```python
from build123d import *
from build123d.topology import SkipClean

# Parameters (mm, degrees)
FILLET_1_R = 2


with BuildPart() as part:
    # ｽｹｯﾁ1 → 回転1 (revolve)
    with SkipClean():  # the faces are left unmerged after this step: merging them gives an invalid solid
        with BuildSketch(Plane.XY, mode=Mode.PRIVATE) as revolve_1_sk:
            with BuildLine():
                ThreePointArc((41.145537471, 23.155045442), (38.343164799, 26.082487024), (34.436430544, 27.159814398))
                Line((34.436430544, 27.159814398), (34.436430544, 11.915416826))
                ThreePointArc((34.436430544, 11.915416826), (39.826138993, 14.147907163), (42.05862933, 19.537615612))
                ThreePointArc((42.05862933, 19.537615612), (41.826831785, 21.403060285), (41.145537471, 23.155045442))
            make_face()
            with BuildLine():
                Line((34.436430544, 11.915416826), (34.436430544, 27.159814398))
                ThreePointArc((34.436430544, 27.159814398), (26.814231757, 19.537615612), (34.436430544, 11.915416826))
            make_face()
            with BuildLine():
                ThreePointArc((42.05862933, 19.537615612), (39.826138993, 14.147907163), (34.436430544, 11.915416826))
                Line((34.436430544, 11.915416826), (34.436430544, 7.442165664))
                Line((34.436430544, 7.442165664), (34.436430544, 4.442165664))
                Line((34.436430544, 4.442165664), (36.436430544, 4.442165664))
                Line((36.436430544, 4.442165664), (36.436430544, 7.442165664))
                Line((36.436430544, 7.442165664), (41.127456758, 7.442165664))
                Line((41.127456758, 7.442165664), (41.127456758, 11.596223188))
                Line((41.127456758, 11.596223188), (44.380435509, 16.421475002))
                Line((44.380435509, 16.421475002), (44.380435509, 22.787256507))
                Line((44.380435509, 22.787256507), (41.735375917, 24.233678208))
                Line((41.735375917, 24.233678208), (41.145537471, 23.155045442))
                ThreePointArc((41.145537471, 23.155045442), (41.826831785, 21.403060285), (42.05862933, 19.537615612))
            make_face()
        revolve(revolve_1_sk.sketch.rotate(Axis((34.436430544, 27.159814398, 0), (0, -1, 0)), 180), axis=Axis((34.436430544, 27.159814398, 0), (0, -1, 0)))

    # ﾌｨﾚｯﾄ1
    fillet_1_edges = [part.edges().sort_by_distance(p)[0] for p in [
        (44.380435509, 22.787256507, 0),
        (41.127456758, 11.596223188, 0),
    ]]
    fillet(fillet_1_edges, radius=FILLET_1_R)


solid = part.part
```
Can you work these out from the model? Positions are in its coordinate system, mm. A direction names the side the tool comes from. Round coordinates to 2 decimals unless told otherwise and drop trailing zeros. Loops run counter-clockwise (first coordinate to the right, second up) from the corner with the lowest first, then second, coordinate; pieces in that order, holes last. Notation, with made-up numbers: M 41.5,57.5 L 95.5,57.5 A19 cw 95.5,64.5 Z; hole C 36,80.25 d3. An arc over 180 degrees is marked long. Write item = value, one per line. Start each with the question number.
(1) Suppose I cut it at B-B on y = 14.75. Write out the boundary of the cut face in (x, z).
(2) I need wall thicknesses on line 1 along Z through (x, y) = (35.25, 19); line 2 along Y through (x, z) = (30.75, -2); line 3 along X through (y, z) = (10.25, 0.5). Which ranges of each line are inside material? Lowest first, please.
(3) Which directions (+Z, -Z, +X, -X, +Y, -Y) give clear straight access to the entire face, cutting with the end or side of a thin tool? Please do faces 1 (the face through (34, 4.442, 0)), 2 (the face through (36, 7.442, -2)).
(4) I'm going to push flat-ended pins straight in: P1, Ø2, axis at y = 9.5, z = -4, coming from the +X side; P2, Ø2, axis at x = 36, y = 9.5, coming from the +Z side; P3, Ø3, axis at y = 20.5, z = 5.5, coming from the +X side; P4, Ø10, axis at y = 25, z = 3, coming from the +X side. Where does each tip first touch, or does it pass through?
(5) Suppose I cut it at A-A on y = 7.75. Write out the boundary of the cut face in (x, z), plus the area to 3 significant figures.
Answer block:
q1.outline = C 34.44,0 d17.63
q2.line_1 = -9.91 to 9.91
q2.line_2 = 7.44 to 25.9
q2.line_3 = 27.76 to 41.11
q3.face_1 = +Z, -Z, +X, -X, -Y
q3.face_2 = -Y
q4.P1 = 40.42
q4.P2 = 6.67
q4.P3 = 43.54
q4.P4 = 44.38
q5.outline = C 34.44,0 d13.38
q5.area = 141 mm²
